Autodesk Fusion 360 part; units mm, degrees
ref_plane "WorkPlane2" through (0, 0, 2.999) normal (0, 0, 1) x (1, 0, 0)
sketch "Sketch4" plane through (0, 0, 2.999) normal (0, 0, 1) x (1, 0, 0)
  line L0 (92.5002, -5.0854) -> (92.4954, -5.0854)
  line L1 (89.5002, -5.0854) -> (44.5002, -5.0854) construction
  line L2 (44.5002, -5.0854) -> (41.5002, -8.0854) construction
  line L3 (41.5002, -8.0854) -> (41.5002, -80.0854) construction
  line L4 (41.5002, -80.0854) -> (44.5002, -83.0854) construction
  line L5 (44.5002, -83.0854) -> (89.5002, -83.0854) construction
  line L6 (92.5002, -80.0854) -> (92.5002, -8.0854) construction
  line L7 (86.0002, -79.0854) -> (86.0002, -83.0854) construction
  line L8 (86.0002, -79.0854) -> (92.5002, -79.0854) construction
  line L9 (86.0002, -79.0854) -> (45.705, -79.088) construction
  line L10 (45.7002, -79.0828) -> (41.5002, -79.0831) construction
  line L11 (45.7002, -9.088) -> (45.7002, -5.0854) construction
  line L12 (45.7002, -9.088) -> (45.705, -79.088) construction
  line L13 (45.6956, -9.088) -> (85.9956, -9.0854) construction
  line L14 (85.9956, -9.0854) -> (92.5002, -9.0854) construction
  line L15 (85.9956, -9.0854) -> (85.9956, -5.0854) construction
  line L16 (85.9956, -79.0854) -> (85.9931, -9.0854) construction
  line L17 (92.5002, -80.0854) -> (89.5002, -83.0854) construction
  line L18 (92.5002, -8.0854) -> (89.5002, -5.0854) construction
  line L19 (44.583, -82.8854) -> (89.4174, -82.8854)
  line L20 (92.3002, -80.0026) -> (89.4174, -82.8854)
  line L21 (92.3002, -80.0026) -> (92.3002, -8.1683)
  line L22 (92.3002, -8.1683) -> (89.4174, -5.2854)
  line L23 (89.4174, -5.2854) -> (44.583, -5.2854)
  line L24 (44.583, -5.2854) -> (41.7002, -8.1683)
  line L25 (41.7002, -8.1683) -> (41.7002, -80.0026)
  line L26 (41.7002, -80.0026) -> (44.583, -82.8854)
  circle A0 centre (85.9956, -9.0854) radius 1.9
  circle A1 centre (45.7002, -9.088) radius 1.9
  circle A2 centre (85.9956, -79.0854) radius 1.9
  circle A3 centre (45.7002, -79.0828) radius 1.9
  line L27 (92.5002, -44.0854) -> (41.5002, -44.0854) construction
  point P0 (92.5002, -83.0854)
  point P1 (92.5002, -5.0854)
  dimension "d34" = 6.5
  dimension "d35" = 4
  dimension "d36" = 4.2
  dimension "d37" = 40.2952
  dimension "d38" = 4
  dimension "d39" = 3
  dimension "d40" = 3
  dimension "d43" = 78
  dimension "d44" = 3
  dimension "d45" = 3
  dimension "d46" = 3
  dimension "d47" = 3
  dimension "d48" = 3
  dimension "d49" = 3
  dimension "d50" = -0.2
  dimension "d53" = 3.8
  dimension "d54" = 3.8
  dimension "d55" = 3.8
  dimension "d56" = 3.8
  dimension "d57" = 51
extrude "Extrude11" add sketch "Sketch4" against normal blind 2
equation "d39 = d40"
equation "d40 = d44"
equation "d45 = d44"
equation "d46 = d44"
equation "d47 = d46"
equation "d48 = d44"
equation "d49 = d48"
equation "d53 = d55"
equation "d54 = d55"
equation "d56 = d55"
The model under review builds one solid part; all positions refer to its coordinate system, in mm. Coordinates: 2 decimals unless noted, no trailing zeros. Write each loop counter-clockwise with the first axis right and the second up, starting at its lowest first coordinate (ties: lowest second). Pieces come first, ordered by that corner, then holes.
1) To check wall thickness, follow probe 1 along X at (y, z) = (-78, 2.7). State the ranges of the line that lie inside material, in increasing order.
2) We need section A-A on z = 1.75. State the section outline as (x, y) points, then the cut area to 3 significant figures.
3) The part is to be moulded in two halves that separate along X. For faces 1 (the face through (43.802, -9.004, 2.013)), 2 (the face through (67, -44, 0.999)), 3 (the face through (90.88, -6.75, 2.01)), say which applies: pulls with the +X half, pulls with the -X half, needs draft (parallel to the pull), parting line crosses it, or undercut.
4) Clearance check with a flat-ended pin moving along its axis: pin 1 Ø5 at (x, y) = (86, -9.09) entering from -Z. State where the tip first meets the part, or that it passes through.
Answer list:
1. probe 1: x = 41.7 to 44.14, 47.26 to 84.44, 87.56 to 92.3
2. outline: (41.7, -80) - (44.58, -82.89) - (89.42, -82.89) - (92.3, -80) - (92.3, -8.17) - (89.42, -5.29) - (44.58, -5.29) - (41.7, -8.17) - close; hole circle Ø3.8 at (45.7, -79.08); hole circle Ø3.8 at (45.7, -9.09); hole circle Ø3.8 at (86, -79.09); hole circle Ø3.8 at (86, -9.09)
2. area: 3,860 mm2
3. face 1: undercut
3. face 2: needs draft
3. face 3: pulls with the +X half
4. pin 1: stops at z = 1
